from build123d import *

# Parameters (mm, degrees)
SKETCH_1_R          = 1.5
SKETCH_1_R_2        = 20
SKETCH_1_R_3        = 2.5
SKETCH_1_R_4        = 10
EXTRUDE_2_DEPTH     = 3
SKETCH_2_R          = 1
SKETCH_2_R_2        = 3.5
CUT_EXTRUDE_1_DEPTH = 3
SKETCH_3_R          = 1.5
CUT_EXTRUDE_2_DEPTH = 10


with BuildPart() as part:
    # 草圖1 → 填料-伸長2 (new body)
    with BuildSketch(Plane(origin=(0, 0, 0), x_dir=(1, 0, 0), z_dir=(0, 1, 0))):
        with BuildLine():
            ThreePointArc((-53.033008589, 53.033008589), (-22.961005942, 55.432771951), (0, 75))
            ThreePointArc((0, 75), (22.961005942, 55.432771951), (53.033008589, 53.033008589))
            ThreePointArc((53.033008589, 53.033008589), (55.432771951, 22.961005942), (75, 0))
            ThreePointArc((75, 0), (55.432771951, -22.961005942), (53.033008589, -53.033008589))
            ThreePointArc((53.033008589, -53.033008589), (22.961005942, -55.432771951), (0, -75))
            ThreePointArc((0, -75), (-22.961005942, -55.432771951), (-53.033008589, -53.033008589))
            ThreePointArc((-53.033008589, -53.033008589), (-55.432771951, -22.961005942), (-75, 0))
            ThreePointArc((-75, 0), (-55.432771951, 22.961005942), (-53.033008589, 53.033008589))
        make_face()
        with Locations(Location((-42.426406871, 42.426406871, 0), (0, 0, 270))):
            Circle(SKETCH_1_R, mode=Mode.SUBTRACT)
        with Locations(Location((-28.991378029, 28.991378029, 0), (0, 0, 270))):
            Circle(SKETCH_1_R, mode=Mode.SUBTRACT)
        with Locations(Location((28.991378029, -28.991378029, 0), (0, 0, 270))):
            Circle(SKETCH_1_R, mode=Mode.SUBTRACT)
        with Locations(Location((42.426406871, -42.426406871, 0), (0, 0, 270))):
            Circle(SKETCH_1_R, mode=Mode.SUBTRACT)
        with Locations(Location((42.426406871, 42.426406871, 0), (0, 0, 270))):
            Circle(SKETCH_1_R, mode=Mode.SUBTRACT)
        with Locations(Location((28.991378029, 28.991378029, 0), (0, 0, 270))):
            Circle(SKETCH_1_R, mode=Mode.SUBTRACT)
        with Locations(Location((-28.991378029, -28.991378029, 0), (0, 0, 270))):
            Circle(SKETCH_1_R, mode=Mode.SUBTRACT)
        with Locations(Location((-42.426406871, -42.426406871, 0), (0, 0, 270))):
            Circle(SKETCH_1_R, mode=Mode.SUBTRACT)
        with Locations(Location((0, 0, 0), (0, 0, 270))):
            Circle(SKETCH_1_R_2, mode=Mode.SUBTRACT)
        with Locations(Location((0, 31.819805153, 0), (0, 0, 270))):
            Circle(SKETCH_1_R, mode=Mode.SUBTRACT)
        with Locations(Location((31.819805153, 0, 0), (0, 0, 270))):
            Circle(SKETCH_1_R, mode=Mode.SUBTRACT)
        with Locations(Location((22.5, 22.5, 0), (0, 0, 270))):
            Circle(SKETCH_1_R, mode=Mode.SUBTRACT)
        with Locations(Location((0, -31.819805153, 0), (0, 0, 270))):
            Circle(SKETCH_1_R, mode=Mode.SUBTRACT)
        with Locations(Location((-22.5, -22.5, 0), (0, 0, 270))):
            Circle(SKETCH_1_R, mode=Mode.SUBTRACT)
        with Locations(Location((-31.819805153, 0, 0), (0, 0, 270))):
            Circle(SKETCH_1_R, mode=Mode.SUBTRACT)
        with Locations(Location((-22.5, 22.5, 0), (0, 0, 270))):
            Circle(SKETCH_1_R, mode=Mode.SUBTRACT)
        with Locations(Location((22.5, -22.5, 0), (0, 0, 270))):
            Circle(SKETCH_1_R, mode=Mode.SUBTRACT)
        with Locations(Location((-21.04758878, 50.813374288, 0), (0, 0, 270))):
            Circle(SKETCH_1_R_3, mode=Mode.SUBTRACT)
        with Locations(Location((21.04758878, 50.813374288, 0), (0, 0, 270))):
            Circle(SKETCH_1_R_3, mode=Mode.SUBTRACT)
        with Locations(Location((50.813374288, 21.04758878, 0), (0, 0, 270))):
            Circle(SKETCH_1_R_3, mode=Mode.SUBTRACT)
        with Locations(Location((50.813374288, -21.04758878, 0), (0, 0, 270))):
            Circle(SKETCH_1_R_3, mode=Mode.SUBTRACT)
        with Locations(Location((21.04758878, -50.813374288, 0), (0, 0, 270))):
            Circle(SKETCH_1_R_3, mode=Mode.SUBTRACT)
        with Locations(Location((-21.04758878, -50.813374288, 0), (0, 0, 270))):
            Circle(SKETCH_1_R_3, mode=Mode.SUBTRACT)
        with Locations(Location((-50.813374288, -21.04758878, 0), (0, 0, 270))):
            Circle(SKETCH_1_R_3, mode=Mode.SUBTRACT)
        with Locations(Location((-50.813374288, 21.04758878, 0), (0, 0, 270))):
            Circle(SKETCH_1_R_3, mode=Mode.SUBTRACT)
        with Locations(Location((0, 50, 0), (0, 0, 270))):
            Circle(SKETCH_1_R_4, mode=Mode.SUBTRACT)
        with Locations(Location((0, -50, 0), (0, 0, 270))):
            Circle(SKETCH_1_R_4, mode=Mode.SUBTRACT)
        with BuildLine():
            Line((-24.409902577, 7.5), (-24.409902577, -7.5))
            ThreePointArc((-24.409902577, -7.5), (-25.909902577, -9), (-27.409902577, -7.5))
            Line((-27.409902577, -7.5), (-27.409902577, 7.5))
            ThreePointArc((-27.409902577, 7.5), (-25.909902577, 9), (-24.409902577, 7.5))
        make_face(mode=Mode.SUBTRACT)
        with BuildLine():
            Line((27.409902577, 7.5), (27.409902577, -7.5))
            ThreePointArc((27.409902577, -7.5), (25.909902577, -9), (24.409902577, -7.5))
            Line((24.409902577, -7.5), (24.409902577, 7.5))
            ThreePointArc((24.409902577, 7.5), (25.909902577, 9), (27.409902577, 7.5))
        make_face(mode=Mode.SUBTRACT)
    extrude(amount=EXTRUDE_2_DEPTH)

    # 草圖2 → 除料-伸長1 (cut)
    with BuildSketch(Plane(origin=(0, 3, 0), x_dir=(1, 0, 0), z_dir=(0, 1, 0))):
        with Locations(Location((-55, 9, 0), (0, 0, 270))):
            Circle(SKETCH_2_R)
        with Locations(Location((-55, -9, 0), (0, 0, 270))):
            Circle(SKETCH_2_R)
        with Locations(Location((55, 9, 0), (0, 0, 270))):
            Circle(SKETCH_2_R)
        with Locations(Location((55, -9, 0), (0, 0, 270))):
            Circle(SKETCH_2_R)
        with Locations(Location((-55, 0, 0), (0, 0, 270))):
            Circle(SKETCH_2_R_2)
        with Locations(Location((55, 0, 0), (0, 0, 270))):
            Circle(SKETCH_2_R_2)
    extrude(amount=-CUT_EXTRUDE_1_DEPTH, mode=Mode.SUBTRACT)

    # 草圖3 → 除料-伸長2 (cut)
    with BuildSketch(Plane(origin=(0, 3, 0), x_dir=(1, 0, 0), z_dir=(0, 1, 0))):
        with Locations(Location((-42.5, 35, 0), (0, 0, 270))):
            Circle(SKETCH_3_R)
        with Locations(Location((42.5, 35, 0), (0, 0, 270))):
            Circle(SKETCH_3_R)
        with Locations(Location((42.5, -35, 0), (0, 0, 270))):
            Circle(SKETCH_3_R)
        with Locations(Location((-42.5, -35, 0), (0, 0, 270))):
            Circle(SKETCH_3_R)
    extrude(amount=-CUT_EXTRUDE_2_DEPTH, mode=Mode.SUBTRACT)


solid = part.part
Design review of the part built by this model. Coordinates are the model's own, in mm. Coordinates: 2 decimals unless noted, no trailing zeros. Order: outer loops, then holes, each group sorted by start corner. A loop starts at its lowest first (then second) coordinate and runs counter-clockwise, first axis right, second up. Notation, with made-up numbers: (59, -16) -> (101, -16) arc R22 cw to (101, 22) -> close; hole circle Ø8 at (-27.5, 78.5). An arc over 180 degrees is marked (long way). One line per item, written item: value.
1) We need section B-B, the plane x = -39. Give the boundary of the cut face in (y, z), then the cut area to 3 significant figures.
Output values:
outline: (0, -51.78) -> (3, -51.78) -> (3, 51.78) -> (0, 51.78) -> close
area: 311 mm2
2) Draft analysis for pull direction Z (two halves, no side actions). For faces 1 (the face through (48.37, 1.48, 20.51)), 2 (the face through (-22.565, 1.479, 55.599)), 3 (the face through (55.27, 1.48, -23.36)), 4 (the face through (18, 3, -18)), state which applies: +Z half, -Z half, draft (parallel to the pull), parting line (faces both ways), or undercut.
Output values:
face 1: undercut
face 2: +Z half
face 3: undercut
face 4: draft
3) We need section A-A, the plane x = 13.5. Give the boundary of the cut face in (y, z).
Output values:
outline: (0, -60.64) -> (3, -60.64) -> (3, -14.76) -> (0, -14.76) -> close; (0, 14.76) -> (3, 14.76) -> (3, 60.64) -> (0, 60.64) -> close
4) Clearance check with flat-ended pins moving along their axes: P1, Ø2.5, axis at x = 42.5, z = -35, coming from the +Y side; P2, Ø2.5, axis at x = -55, z = 9, coming from the +Y side; P3, Ø0.9, axis at y = 2, z = 1.5, coming from the +X side. State where each tip first meets the part, or that it passes through.
Output values:
P1: passes through
P2: stops at y = 3
P3: stops at x = 73.37
5) We need section C-C, the plane y = 1. Count the separate pieces of the cut face and the enclosed holes in it, then the cut area to 3 significant figures.
Output values:
separate pieces: 1
enclosed holes: 39
area: 10,600 mm2
6) To check wall thickness, follow probe 1 along X at (y, z) = (1.5, 49.5); probe 2 along X at (y, z) = (1.35, 35); probe 3 along X at (y, z) = (2.25, 43). State the ranges of each line that lie inside material, in increasing order. Write a range as [from, to].
Output values:
probe 1: x = [-52.33, -23.17], [-18.92, -9.99], [9.99, 18.92], [23.17, 52.33]
probe 2: x = [-52.17, -44], [-41, 41], [44, 52.17]
probe 3: x = [-51.72, -43.81], [-41.04, -7.14], [7.14, 41.04], [43.81, 51.72]
